Geometry check sheet. Reference: the model listing, model coordinates, mm. A direction names the side the tool comes from. Give positions to 0.01 mm unless a question says otherwise; leave off trailing zeros. Order: outer loops, then holes, each group sorted by start corner. A loop starts at its lowest first (then second) coordinate and runs counter-clockwise, first axis right, second up.
from build123d import *

# Parameters (mm, degrees)
SKETCH2_R           = 35
SKETCH2_R_2         = 33
BOSS_EXTRUDE1_DEPTH = 39
BOSS_EXTRUDE2_START = -2
SKETCH3_R           = 35
BOSS_EXTRUDE2_DEPTH = 2
SKETCH7_R           = 5.5
SKETCH7_R_2         = 1.5
SKETCH7_R_3         = 4
BOSS_EXTRUDE4_DEPTH = 19
SKETCH8_R           = 3
CUT_EXTRUDE3_DEPTH  = 15
CHAMFER1_SIZE       = 3
SKETCH9_R           = 15
SKETCH9_R_2         = 14
CUT_EXTRUDE4_DEPTH  = 0.5
SKETCH10_R          = 1.5
SKETCH11_R          = 8
CUT_EXTRUDE5_DEPTH  = 87.396599101
SKETCH12_R          = 10
SKETCH12_R_2        = 8
BOSS_EXTRUDE5_DEPTH = 15
SKETCH13_R          = 55
SKETCH13_R_2        = 35
CUT_EXTRUDE6_DEPTH  = 64.01587119
FILLET1_R           = 10


with BuildPart() as part:
    # Sketch2 → Boss-Extrude1 (new body)
    with BuildSketch(Plane(origin=(0, 31.812232957, 0), x_dir=(1, 0, 0), z_dir=(0, 1, 0))):
        Circle(SKETCH2_R)
        Circle(SKETCH2_R_2, mode=Mode.SUBTRACT)
    extrude(amount=BOSS_EXTRUDE1_DEPTH)

    # Sketch3 → Boss-Extrude2 (add)
    with BuildSketch(Plane(origin=(0, 70.812232957, 0), x_dir=(1, 0, 0), z_dir=(0, 1, 0)).offset(BOSS_EXTRUDE2_START)):
        Circle(SKETCH3_R)
    extrude(amount=BOSS_EXTRUDE2_DEPTH)

    # Sketch7 → Boss-Extrude4 (add)
    # profile 1 of 2: a face of its own
    with BuildSketch(Plane.XZ.offset(-68.812232957)):
        with Locations(Location((25, 0, 0), (0, 0, 180))):
            Circle(SKETCH7_R)
        with Locations((25, 0)):
            Circle(SKETCH7_R_2, mode=Mode.SUBTRACT)
    # profile 2 of 2: a face of its own
    with BuildSketch(Plane.XZ.offset(-68.812232957)):
        with Locations(Location((-25, 0, 0), (0, 0, 180))):
            Circle(SKETCH7_R_3)
        with Locations((-25, 0)):
            Circle(SKETCH7_R_2, mode=Mode.SUBTRACT)
    extrude(amount=BOSS_EXTRUDE4_DEPTH)

    # Sketch8 → Cut-Extrude3 (cut)
    with BuildSketch(Plane(origin=(0, 70.812232957, 0), x_dir=(1, 0, 0), z_dir=(0, 1, 0))):
        with Locations(Location((25, 0, 0), (0, 0, 180))):
            Circle(SKETCH8_R)
        with Locations(Location((-25, 0, 0), (0, 0, 180))):
            Circle(SKETCH8_R)
    extrude(amount=-CUT_EXTRUDE3_DEPTH, mode=Mode.SUBTRACT)

    # Chamfer1
    # the kernel refuses this chamfer: 3 mm, written as the material it adds along each edge
    with BuildSketch(Plane(origin=(0, 68.812232957, 0), x_dir=(1, 0, 0), z_dir=(0, 0, -1))) as chamfer1_piece_1:
        Polygon((33, CHAMFER1_SIZE), (33 - CHAMFER1_SIZE, 0), (33, 0), align=None)
    revolve(axis=Axis((0, 68.812232957, 0), (0, -1, 0)))

    # Sketch9 → Cut-Extrude4 (cut)
    with BuildSketch(Plane(origin=(0, 70.812232957, 0), x_dir=(1, 0, 0), z_dir=(0, 1, 0))):
        with Locations(Location((0, 0, 0), (0, 0, 180))):
            Circle(SKETCH9_R)
        with Locations(Location((0, 0, 0), (0, 0, 180))):
            Circle(SKETCH9_R_2, mode=Mode.SUBTRACT)
    extrude(amount=-CUT_EXTRUDE4_DEPTH, mode=Mode.SUBTRACT)

    # Sketch10 → Cut-Revolve1 (revolve, cut)
    with BuildSketch(Plane.XY, mode=Mode.PRIVATE) as cut_revolve1_sk:
        with Locations((35, 34.312232957)):
            Circle(SKETCH10_R)
    revolve(cut_revolve1_sk.sketch.rotate(Axis((0, 31.812232957, 0), (0, 1, 0)), 4.795108108), axis=Axis((0, 31.812232957, 0), (0, 1, 0)), mode=Mode.SUBTRACT)

    # Sketch11 → Cut-Extrude5 (cut, through all)
    with BuildSketch(Plane(origin=(0, 0, 0), x_dir=(0, 0, -1), z_dir=(1, 0, 0))):
        with Locations(Location((14.5, 49.812232957, 0), (0, 0, 180))):
            Circle(SKETCH11_R)
        with Locations(Location((-14.5, 49.812232957, 0), (0, 0, 180))):
            Circle(SKETCH11_R)
    extrude(amount=CUT_EXTRUDE5_DEPTH, mode=Mode.SUBTRACT)

    # Sketch12 → Boss-Extrude5 (add)
    # profile 1 of 4: a face of its own
    with BuildSketch(Plane(origin=(20, 0, 0), x_dir=(0, 0, -1), z_dir=(1, 0, 0))):
        with BuildLine():
            Line((-27.5, 70.812232957), (-24.5, 49.812232957))
            ThreePointArc((-24.5, 49.812232957), (-14.5, 59.812232957), (-4.5, 49.812232957))
            Line((-4.5, 49.812232957), (-4.5, 70.812232957))
            Line((-4.5, 70.812232957), (-27.5, 70.812232957))
        make_face()
    # profile 2 of 4: a face of its own
    with BuildSketch(Plane(origin=(20, 0, 0), x_dir=(0, 0, -1), z_dir=(1, 0, 0))):
        with Locations((-14.5, 49.812232957)):
            Circle(SKETCH12_R)
        with Locations((-14.5, 49.812232957)):
            Circle(SKETCH12_R_2, mode=Mode.SUBTRACT)
    # profile 3 of 4: a face of its own
    with BuildSketch(Plane(origin=(20, 0, 0), x_dir=(0, 0, -1), z_dir=(1, 0, 0))):
        with Locations((14.5, 49.812232957)):
            Circle(SKETCH12_R)
        with Locations((14.5, 49.812232957)):
            Circle(SKETCH12_R_2, mode=Mode.SUBTRACT)
    # profile 4 of 4: a face of its own
    with BuildSketch(Plane(origin=(20, 0, 0), x_dir=(0, 0, -1), z_dir=(1, 0, 0))):
        with BuildLine():
            ThreePointArc((4.5, 49.812232957), (14.5, 59.812232957), (24.5, 49.812232957))
            Line((24.5, 49.812232957), (27.5, 70.812232957))
            Line((27.5, 70.812232957), (4.5, 70.812232957))
            Line((4.5, 70.812232957), (4.5, 49.812232957))
        make_face()
    extrude(amount=BOSS_EXTRUDE5_DEPTH)

    # Sketch13 → Cut-Extrude6 (cut, through all)
    with BuildSketch(Plane(origin=(0, 70.812232957, 0), x_dir=(1, 0, 0), z_dir=(0, 1, 0))):
        Circle(SKETCH13_R)
        Circle(SKETCH13_R_2, mode=Mode.SUBTRACT)
    extrude(amount=-CUT_EXTRUDE6_DEPTH, mode=Mode.SUBTRACT)

    # Fillet1
    # the kernel refuses this fillet: 10 mm, written as the material it adds along each edge
    with BuildSketch(Plane(origin=(-25, 68.812232957, 0), x_dir=(-1, 0, 0), z_dir=(0, 0, 1))) as fillet1_piece_1_section:
        with BuildLine():
            CenterArc((4 + FILLET1_R, FILLET1_R), FILLET1_R, 180, 90)
            Line((4 + FILLET1_R, 0), (4, 0))
            Line((4, 0), (4, FILLET1_R))
        make_face()
    fillet1_piece_1 = revolve(axis=Axis((-25, 68.812232957, 0), (0, -1, 0)), mode=Mode.PRIVATE)
    fillet1_piece_1 = fillet1_piece_1 & Plane(origin=(0, 65.946902584, 0), x_dir=(1, 0, 0), z_dir=(0, -1, 0)) * Cylinder(35, 56, mode=Mode.PRIVATE)
    add(fillet1_piece_1)


solid = part.part
Item 1: Gauge pin test, flat ends, axial feed: pin 1 (1.8 mm diameter, centred on x = 24.5, z = -1, fed in from +Y); pin 2 (24 mm diameter, centred on x = 0, z = 0, fed in from -Y); pin 3 (17.5 mm diameter, centred on y = 58.5, z = 17, fed in from -X); pin 4 (2.5 mm diameter, centred on x = 25, z = 0, fed in from +Y). Record the tip position at first contact, or that the pin passes through.
Reported:
pin 1: stops at y = 55.81
pin 2: stops at y = 68.76
pin 3: stops at x = -34.01
pin 4: passes through
Item 2: Draft check along X on faces 1 (the flat face through (0, 70.812, 0)), 2 (the flat face through (29, 68.812, -4)), 3 (the cylindrical face through (-7.587, 32.305, 34.168)). Enter one of: released by +X, released by -X, zero draft, split by the parting line, or undercut.
Reported:
face 1: zero draft
face 2: undercut
face 3: split by the parting line
Item 3: Set-up check for faces 4 (the flat face through (26.3, 49.812, -1.1)), 5 (the cylindrical face through (-22, 63, 0)), 6 (the cylindrical face through (-34.966, 53.557, -1.539)): record each of +Z, -Z, +X, -X, +Y, -Y from which the full face is reachable in a straight line by a thin tool's end or side.
Reported:
face 4: -Y
face 5: +Y
face 6: +Y, -Y
Item 4: Sectioned sample at D-D (y = 38.5). Enter the section's corners in (x, z), and give its area (3 significant figures).
Reported:
outline: circle Ø70 at (0, 0); hole circle Ø66 at (0, 0)
area: 427 mm2
Item 5: Sectioned sample at C-C (x = 25). Give the number of separate pieces and of enclosed holes in the cut face, and give its area (3 significant figures).
Reported:
separate pieces: 2
enclosed holes: 2
area: 900 mm2
Item 6: Sectioned sample at B-B (x = 0). Enter the section's corners in (y, z).
Reported:
outline: (31.81, -35) - (32.81, -35) arc R1.5 cw to (35.81, -35) - (70.81, -35) - (70.81, -15) - (70.31, -15) - (70.31, -14) - (70.81, -14) - (70.81, 14) - (70.31, 14) - (70.31, 15) - (70.81, 15) - (70.81, 35) - (35.81, 35) arc R1.5 cw to (32.81, 35) - (31.81, 35) - (31.81, 33) - (65.81, 33) - (68.81, 30) - (68.81, -30) - (65.81, -33) - (31.81, -33) - close
Item 7: Sectioned sample at A-A (y = 64.5). Enter the section's corners in (x, z), and give its area (3 significant figures).
Reported:
outline: circle Ø70 at (0, 0); circle Ø11.55 at (-25, 0); hole circle Ø6 at (-25, 0); hole (20, -26.25) - (20, -4.5) - (21.84, -4.5) arc R5.5 cw to (21.84, 4.5) - (20, 4.5) - (20, 26.25) arc R33 ccw (long way) to start; hole circle Ø6 at (25, 0); hole (28.16, -4.5) - (32.69, -4.5) arc R33 ccw to (32.69, 4.5) - (28.16, 4.5) arc R5.5 cw to start
area: 922 mm2
Item 8: Scan lines: L1, parallel to X at y = 51, z = 0; L2, parallel to Z at x = -1, y = 46.5; L3, parallel to Y at x = 29, z = 14. Record each from-to range of solid material in increasing order.
Reported:
L1: x = -35 to -33, -29 to -26.5, -23.5 to -21, 19.5 to 23.5, 26.5 to 30.5, 33 to 35
L2: z = -34.99 to -32.98, 32.98 to 34.99
L3: y = 39.82 to 41.83, 57.8 to 70.81
